from build123d import *

# Parameters (mm, degrees)
SKETCH039_W             = 110
SKETCH039_H             = 60
PAD024_DEPTH            = 5
SKETCH040_W             = 10
SKETCH040_H             = 10
PAD025_DEPTH            = 90
SKETCH041_W             = 4.8
SKETCH041_H             = 4.8
PAD026_DEPTH            = 100
SKETCH042_R             = 10
POCKET015_DEPTH         = 3.5
FILLET002_R             = 25
BODY013_PITCH_ANGLE     = 70
BODY013_PLACEMENT_ANGLE = 90


with BuildPart() as part:
    # Sketch039 → Pad024 (new body)
    with BuildSketch(Plane.XY.offset(-2.5)):
        with Locations((52.5, 0)):
            Rectangle(SKETCH039_W, SKETCH039_H)
    extrude(amount=PAD024_DEPTH)

    # Sketch040 → Pad025 (join, symmetric)
    with BuildSketch(Plane.XZ):
        with Locations((2.5, 2.5)):
            Rectangle(SKETCH040_W, SKETCH040_H)
        with Locations((62.5, 2.5)):
            Rectangle(SKETCH040_W, SKETCH040_H)
    extrude(amount=PAD025_DEPTH, both=True)

    # Sketch041 → Pad026 (join, symmetric)
    with BuildSketch(Plane.XZ):
        with Locations((2.4, 2.4)):
            Rectangle(SKETCH041_W, SKETCH041_H)
        with Locations((62.4, 2.4)):
            Rectangle(SKETCH041_W, SKETCH041_H)
    extrude(amount=PAD026_DEPTH, both=True)

    # Sketch042 → Pocket015 (cut, symmetric)
    with BuildSketch(Plane.XY):
        with Locations((32.5, 0)):
            Circle(SKETCH042_R)
        with Locations((85, 0)):
            Circle(SKETCH042_R)
    extrude(amount=POCKET015_DEPTH, both=True, mode=Mode.SUBTRACT)

    # Fillet002
    fillet002_edges = [part.edges().sort_by_distance(p)[0] for p in [
        (107.5, 30, 0),
        (107.5, -30, 0),
    ]]
    fillet(fillet002_edges, radius=FILLET002_R)


with BuildPart() as part_1:
    # Body013 pitch: moved
    add(part.part.rotate(Axis((0, 0, 0), (0, 1, 0)), BODY013_PITCH_ANGLE))


with BuildPart() as part_2:
    # Body013 placement: moved
    add(part_1.part.moved(Location((75.5, 0.18654, -53.140994))).rotate(Axis((75.5, 0.18654, -53.140994), (0, 0, 1)), BODY013_PLACEMENT_ANGLE))


solid = part_2.part
Input: part model. Units: mm. Frame: model coordinates. A direction names the side the tool comes from. Give positions to 0.01 mm unless a question says otherwise; leave off trailing zeros. Loops run counter-clockwise (first coordinate to the right, second up) from the corner with the lowest first, then second, coordinate; pieces in that order, holes last. Notation, with made-up numbers: (31.25, 78.25) - (35.25, 78.25) arc R25 ccw to (35.25, 99.25) - close; hole circle Ø10 at (52, 64). An arc over 180 degrees is marked (long way). Use CSV: the item, a comma, the result in double quotes. Start each with the question number.
Item 1: Line query: line 1 (X direction, y = 21, z = -115.5); line 2 (X direction, y = 31, z = -138); line 3 (Y direction, x = 84, z = -126). Output: solid intervals per line, ascending.
Item 2: Section B-B on x = 73. Return loops of the section in (y, z).
Item 3: Reachability of faces 1 (the flat face through (76.76, 26.6, -115.36)), 2 (the flat face through (170.43, 2.41, -52.33)), 3 (the flat face through (75.08, 35.407, -142.599)), 4 (the flat face through (-14.5, 27, -110)), 5 (the flat face through (-19.57, 0.996, -55.365)) from +Z, -Z, +X, -X, +Y, -Y: full face, straight path, thin tool, end or side. Return the list, or none.
Item 4: Section A-A on x = 148. Return loops of the section in (y, z), then the cut area to 3 significant figures.
Item 5: Contact query for flat-ended pins moving along their axis: P1, Ø10, axis at y = 16, z = -80.5, coming from the +X side; P2, Ø5, axis at y = 23.5, z = -125, coming from the -X side; P3, Ø1.5, axis at x = 70.5, z = -69.5, coming from the -Y side. Output: stop coordinate, or through.
Item 6: Mould query, pull axis Y, two halves, no side actions, for faces 6 (the flat face through (76.76, 23.18, -105.962)), 7 (the flat face through (-24.5, 24, -111)), 8 (the flat face through (170.43, 4.052, -56.842)), 9 (the flat face through (76.76, 1.615, -49.961)). Classes: pulls with the +Y half, pulls with the -Y half, needs draft (parallel to the pull), parting line crosses it, or undercut.
Ans:
1,line 1,"x = -14.5 to 165.5"
1,line 2,"x = 46.74 to 67.01, 83.99 to 104.26"
1,line 3,"y = 24.04 to 29.37"
2,outline,"(-3.02, -51.65) - (5.64, -75.44) - (10.34, -73.73) - (5.1, -59.33) - (9.8, -57.62) - (6.38, -48.23) - close; (12.26, -93.63) - (23.6, -124.77) - (28.3, -123.06) - (25.62, -115.72) - (30.32, -114.01) - (26.9, -104.61) - (22.2, -106.32) - (16.96, -91.92) - close; (30.22, -142.97) - (34.6, -155.01) - (39.3, -153.3) - (34.92, -141.26) - close"
3,face 1,"+Y"
3,face 2,"+Z, +X, -Y"
3,face 3,"+X, -X, +Y"
3,face 4,"-X"
3,face 5,"-Z, -X, -Y"
4,outline,"(-3.02, -51.65) - (0.4, -61.04) - (9.8, -57.62) - (6.38, -48.23) - close; (17.5, -108.03) - (20.92, -117.43) - (30.32, -114.01) - (26.9, -104.61) - close"
4,area,"200 mm2"
5,P1,"stops at x = 105.5"
5,P2,"stops at x = 45.5"
5,P3,"stops at y = 3.21"
6,face 6,"undercut"
6,face 7,"needs draft"
6,face 8,"pulls with the +Y half"
6,face 9,"pulls with the -Y half"
